For this review, take the finished solid that the model builds, in its own axes (mm). Round coordinates to 2 decimals unless told otherwise and drop trailing zeros. Order: outer loops, then holes, each group sorted by start corner. A loop starts at its lowest first (then second) coordinate and runs counter-clockwise, first axis right, second up.
from build123d import *

# Parameters (mm, degrees)
DRAFT1_START       = -9.525
DRAFT1_OUTLINE_R   = 4.838885636
DRAFT1_DEPTH       = 19.05
DRAFT2_ANGLE       = 45
DRAFT3_ANGLE       = 44.810245375
DRAFT4_ANGLE       = 45
DRAFT5_ANGLE       = 45
DRAFT6_ANGLE       = 44.810245375
DRAFT7_ANGLE       = 44.810245375
DRAFT8_ANGLE       = 45
DRAFT9_ANGLE       = 45
DRAFT10_ANGLE      = 45
DRAFT11_ANGLE      = 45
DRAFT12_ANGLE      = 45
FILLET1_R          = 0.0127
CHAMFER1_SIZE      = 0.017960514
FILLET2_R          = 0.3
SKETCH1_R          = 2.54
CUT_EXTRUDE1_DEPTH = 21.241841037


with BuildPart() as part:
    # Draft1: read off the stored shape, not the designer's step
    # Draft1 outline → Draft1 (new body)
    with BuildSketch(Plane.XY.offset(DRAFT1_START)):
        Circle(DRAFT1_OUTLINE_R)
        Polygon((-1.0918, 1.6252), (-0.9521, 1.4855), (-0.9521, 1.6125), (0.9521, 1.6125), (0.9521, 1.4855), (1.0918, 1.6252), (1.168210303, 1.548789697), (1.2315, 1.6125), (1.6125, 1.6125), (1.6125, 1.231499999), (1.485500001, 1.231499999), (1.6252, 1.0918), (1.4855, 0.9521), (1.6125, 0.9521), (1.6125, -0.9521), (1.4855, -0.9521), (1.6252, -1.0918), (1.485500001, -1.231499999), (1.612499999, -1.231499999), (1.6125, -1.6125), (1.2315, -1.6125), (1.2315, -1.4855), (1.0918, -1.6252), (0.9521, -1.4855), (0.9521, -1.6125), (-0.9521, -1.6125), (-0.9521, -1.4855), (-1.0918, -1.6252), (-1.2315, -1.4855), (-1.2315, -1.6125), (-1.6125, -1.6125), (-1.6125, -1.231499999), (-1.485500001, -1.231499999), (-1.6252, -1.0918), (-1.4855, -0.9521), (-1.6125, -0.9521), (-1.6125, 0.9521), (-1.4855, 0.9521), (-1.6252, 1.0918), (-1.485500001, 1.231499999), (-1.612499999, 1.231499999), (-1.6125, 1.6125), (-1.2315, 1.6125), (-1.2315, 1.4855), align=None, mode=Mode.SUBTRACT)
    extrude(amount=DRAFT1_DEPTH)

    # Draft1 2 outline → Draft1 2 (revolve, cut)
    with BuildSketch(Plane.XZ):
        with BuildLine():
            Line((1.6125, -9.525), (4, -9.525))
            ThreePointArc((4, -9.525), (2.809495756, -9.361292288), (1.6125, -9.254982683))
            Line((1.6125, -9.254982683), (1.6125, -9.525))
        make_face()
        with BuildLine():
            Line((1.6125, 9.525), (1.6125, 9.254982683))
            ThreePointArc((1.6125, 9.254982683), (2.809495756, 9.361292288), (4, 9.525))
            Line((4, 9.525), (1.6125, 9.525))
        make_face()
    revolve(axis=Axis((0, 0, 0), (0, 0, 1)), mode=Mode.SUBTRACT)

    # Draft2
    draft2_faces = [part.faces().sort_by_distance(p)[0] for p in [
        (1.549009001, 1.231499999, 0),
    ]]
    draft(draft2_faces, Plane(origin=(1.6125, -1.6125, 11.43), x_dir=(0, 0, -1), z_dir=(-1, 0, 0)), DRAFT2_ANGLE)

    # Draft3
    draft3_faces = [part.faces().sort_by_distance(p)[0] for p in [
        (1.549009001, -1.231499999, 0),
    ]]
    draft(draft3_faces, Plane(origin=(1.6125, -1.6125, 11.43), x_dir=(0, 0, -1), z_dir=(-1, 0, 0)), DRAFT3_ANGLE)

    # Draft4
    draft4_faces = [part.faces().sort_by_distance(p)[0] for p in [
        (1.2315, -1.549009001, 0),
    ]]
    draft(draft4_faces, Plane(origin=(-1.6125, -1.6125, 11.43), x_dir=(0, 0, 1), z_dir=(0, 1, 0)), DRAFT4_ANGLE)

    # Draft5
    draft5_faces = [part.faces().sort_by_distance(p)[0] for p in [
        (-1.2315, 1.549009001, 0),
    ]]
    draft(draft5_faces, Plane(origin=(1.6125, 1.6125, 11.43), x_dir=(0, 0, -1), z_dir=(0, -1, 0)), DRAFT5_ANGLE)

    # Draft6
    draft6_faces = [part.faces().sort_by_distance(p)[0] for p in [
        (-1.549009001, 1.231499999, 0),
    ]]
    draft(draft6_faces, Plane(origin=(-1.6125, 1.6125, 11.43), x_dir=(0, 0, 1), z_dir=(1, 0, 0)), DRAFT6_ANGLE)

    # Draft7
    draft7_faces = [part.faces().sort_by_distance(p)[0] for p in [
        (-1.2315, -1.549009001, 0),
    ]]
    draft(draft7_faces, Plane(origin=(-1.6125, -1.6125, 11.43), x_dir=(0, 0, 1), z_dir=(0, 1, 0)), DRAFT7_ANGLE)

    # Draft8
    draft8_faces = [part.faces().sort_by_distance(p)[0] for p in [
        (-1.549009001, -1.231499999, 0),
    ]]
    draft(draft8_faces, Plane(origin=(-1.6125, 1.6125, 11.43), x_dir=(0, 0, 1), z_dir=(1, 0, 0)), DRAFT8_ANGLE)

    # Draft9
    draft9_faces = [part.faces().sort_by_distance(p)[0] for p in [
        (-0.9521, 1.549009008, 0),
        (0.9521, 1.549009008, 0),
    ]]
    draft(draft9_faces, Plane(origin=(1.6125, 1.6125, 11.43), x_dir=(0, 0, -1), z_dir=(0, -1, 0)), DRAFT9_ANGLE)

    # Draft10
    draft10_faces = [part.faces().sort_by_distance(p)[0] for p in [
        (1.549009008, -0.9521, 0),
        (1.549009008, 0.9521, 0),
    ]]
    draft(draft10_faces, Plane(origin=(1.6125, -1.6125, 11.43), x_dir=(0, 0, -1), z_dir=(-1, 0, 0)), DRAFT10_ANGLE)

    # Draft11
    draft11_faces = [part.faces().sort_by_distance(p)[0] for p in [
        (-0.9521, -1.549009008, 0),
        (0.9521, -1.549009008, 0),
    ]]
    draft(draft11_faces, Plane(origin=(-1.6125, -1.6125, 11.43), x_dir=(0, 0, 1), z_dir=(0, 1, 0)), DRAFT11_ANGLE)

    # Draft12
    draft12_faces = [part.faces().sort_by_distance(p)[0] for p in [
        (-1.549009008, 0.9521, 0),
        (-1.549009008, -0.9521, 0),
    ]]
    draft(draft12_faces, Plane(origin=(-1.6125, 1.6125, 11.43), x_dir=(0, 0, 1), z_dir=(1, 0, 0)), DRAFT12_ANGLE)

    # Fillet1
    fillet1_edges = [part.edges().sort_by_distance(p)[0] for p in [
        (-1.0156, 1.549, 0),
        (-1.168, 1.549, 0),
        (-1.548789698, 1.168210302, 0),
        (-1.549, 1.0156, 0),
        (-1.549, -1.0156, 0),
        (-1.549, -1.168, 0),
        (-1.168210303, -1.548789697, 0),
        (-1.0156, -1.549, 0),
        (1.0156, -1.549, 0),
        (1.168, -1.549, 0),
        (1.548789698, -1.168210302, 0),
        (1.549, -1.0156, 0),
        (1.549, 1.0156, 0),
        (1.549, 1.168, 0),
        (1.168210303, 1.548789697, 0),
        (1.0156, 1.549, 0),
    ]]
    fillet(fillet1_edges, radius=FILLET1_R)

    # Chamfer1
    chamfer1_edges = [part.edges().sort_by_distance(p)[0] for p in [
        (-1.0918, 1.6252, 0),
        (-1.6252, 1.0918, 0),
        (-1.6252, -1.0918, 0),
        (1.6252, -1.0918, 0),
        (1.6252, 1.0918, 0),
        (1.0918, 1.6252, 0),
    ]]
    chamfer(chamfer1_edges, length=CHAMFER1_SIZE)

    # Fillet2
    fillet2_edges = [part.edges().sort_by_distance(p)[0] for p in [
        (-4.838885636, 0, 9.525),
        (-4.838885636, 0, -9.525),
        (-1.6125, 1.6125, 0),
        (-1.6125, -1.6125, 0),
        (1.6125, -1.6125, 0),
        (1.6125, 1.6125, 0),
    ]]
    fillet(fillet2_edges, radius=FILLET2_R)

    # Sketch1 → Cut-Extrude1 (cut, through all)
    with BuildSketch(Plane.XY.offset(9.525)):
        Circle(SKETCH1_R)
    extrude(amount=-CUT_EXTRUDE1_DEPTH, mode=Mode.SUBTRACT)


solid = part.part
(1) Wall thickness on L1, parallel to Y at x = 0, z = 1.25; L2, parallel to X at y = -1.75, z = -4.25; L3, parallel to X at y = -0.25, z = -8: over which ranges is each line inside the solid? List them lowest first.
(2) Draft analysis for pull direction X (two halves, no side actions). For faces 1 (the face through (-0.6, 4.8, -0.1)), 2 (the face through (3, -3, 9.525)), 3 (the face through (-0.33, 2.52, 0.13)), state which applies: pulls with the +X half, pulls with the -X half, needs draft (parallel to the pull), parting line crosses it, or undercut.
(3) Add section C-C on z = 5. Give the boundary of the cut face in (x, y).
(4) Add section A-A on x = 0. Give the boundary of the cut face in (y, z) (3 decimals), plus the area to 3 significant figures.
(5) Clearance check with flat-ended pins moving along their axes: P1, Ø1.5, axis at x = 2.5, z = 2, coming from the -Y side; P2, Ø1, axis at x = 1, z = -2.5, coming from the -Y side; P3, Ø1, axis at x = 1, y = -2, coming from the -Z side. State where each tip first meets the part, or that it passes through.
Here are the results:
1. L1: y = -4.84 to -2.54, 2.54 to 4.84
1. L2: x = -4.51 to -1.84, 1.84 to 4.51
1. L3: x = -4.83 to -2.53, 2.53 to 4.83
2. face 1: parting line crosses it
2. face 2: needs draft
2. face 3: undercut
3. outline: circle Ø9.68 at (0, 0); hole circle Ø5.08 at (0, 0)
4. outline: (-4.839, -9.225) arc R0.3 ccw to (-4.539, -9.525) - (-4, -9.525) arc R25 cw to (-2.54, -9.332) - (-2.54, 9.332) arc R25 cw to (-4, 9.525) - (-4.539, 9.525) arc R0.3 ccw to (-4.839, 9.225) - close; (2.54, -9.332) arc R25 cw to (4, -9.525) - (4.539, -9.525) arc R0.3 ccw to (4.839, -9.225) - (4.839, 9.225) arc R0.3 ccw to (4.539, 9.525) - (4, 9.525) arc R25 cw to (2.54, 9.332) - close
4. area: 86.9 mm2
5. P1: stops at y = -4.51
5. P2: stops at y = -4.81
5. P3: stops at z = -9.35
